Source: CAD feature listing. Evaluate the final solid. Frame: model axes, mm. A direction names the side the tool comes from. Round coordinates to 2 decimals unless told otherwise and drop trailing zeros. Write each loop counter-clockwise with the first axis right and the second up, starting at its lowest first coordinate (ties: lowest second). Pieces come first, ordered by that corner, then holes.
from build123d import *

# Parameters (mm, degrees)
SKETCH1_W               = 38.1
SKETCH1_H               = 19.05
BOSS_EXTRUDE1_DEPTH     = 12.7
SKETCH2_W               = 11.43
SKETCH2_H               = 19.05
CUT_EXTRUDE1_DEPTH      = 20.05
SKETCH3_R               = 3.302
CUT_EXTRUDE2_DEPTH      = 7.35
SKETCH7_R               = 6.35
CUT_EXTRUDE6_DEPTH      = 19.05
F_1_4_20_TAPPED_HOLE2_D = 5.1054


with BuildPart() as part:
    # Sketch1 → Boss-Extrude1 (new body, symmetric)
    with BuildSketch(Plane(origin=(0, 0, 0), x_dir=(1, 0, 0), z_dir=(0, 1, 0))):
        Rectangle(SKETCH1_W, SKETCH1_H)
    extrude(amount=BOSS_EXTRUDE1_DEPTH, both=True)

    # Sketch2 → Cut-Extrude1 (cut, through all)
    with BuildSketch(Plane.XY.offset(9.525)):
        with Locations((-13.335, 3.175)):
            Rectangle(SKETCH2_W, SKETCH2_H)
    cut_extrude1 = extrude(amount=-CUT_EXTRUDE1_DEPTH, mode=Mode.SUBTRACT)

    # Sketch3 → Cut-Extrude2 (cut, through all)
    with BuildSketch(Plane(origin=(0, -6.35, 0), x_dir=(1, 0, 0), z_dir=(0, 1, 0))):
        with Locations((-12.7, 0)):
            Circle(SKETCH3_R)
    cut_extrude2 = extrude(amount=-CUT_EXTRUDE2_DEPTH, mode=Mode.SUBTRACT)

    # Mirror1: Cut-Extrude1, Cut-Extrude2 across plane
    add(cut_extrude1.mirror(Plane(origin=(0, 0, 0), x_dir=(0, 0, 1), z_dir=(1, 0, 0))), mode=Mode.SUBTRACT)
    add(cut_extrude2.mirror(Plane(origin=(0, 0, 0), x_dir=(0, 0, 1), z_dir=(1, 0, 0))), mode=Mode.SUBTRACT)

    # Sketch7 → Cut-Extrude6 (cut)
    with BuildSketch(Plane.XZ.offset(12.7)):
        Circle(SKETCH7_R)
    extrude(amount=-CUT_EXTRUDE6_DEPTH, mode=Mode.SUBTRACT)

    # 1/4-20 Tapped Hole2 (through all)
    with Locations(Plane(origin=(0, 12.7, 0), x_dir=(1, 0, 0), z_dir=(0, 1, 0))):
        with Locations((0, 0)):
            Hole(F_1_4_20_TAPPED_HOLE2_D / 2)


solid = part.part
1) Pull-direction query (Z, two-part tool) for faces 4 (the face through (-2.435, 9.481, -0.767)), 5 (the face through (0, -3, -9.525)), 6 (the face through (19.05, -9, 0)); classes: released by +Z, released by -Z, zero draft, split by the parting line, or undercut.
Taken from the geometry:
face 4: undercut
face 5: released by -Z
face 6: zero draft
2) Section query A-A on x = 0. Return the cut outline in (y, z) (3 decimals), then the cut area to 3 significant figures.
Taken from the geometry:
outline: (-12.7, -9.525) - (12.7, -9.525) - (12.7, -2.553) - (6.35, -2.553) - (6.35, -6.35) - (-12.7, -6.35) - close; (-12.7, 6.35) - (6.35, 6.35) - (6.35, 2.553) - (12.7, 2.553) - (12.7, 9.525) - (-12.7, 9.525) - close
area: 210 mm2
3) Material intervals for line 1 (Z direction, x = 12.7, y = -9.5) (3 decimals); line 2 (Z direction, x = 0, y = 10) (3 decimals); line 3 (Y direction, x = -12, z = -7), sorted ascending.
Taken from the geometry:
line 1: z = -9.525 to -3.302, 3.302 to 9.525
line 2: z = -9.525 to -2.553, 2.553 to 9.525
line 3: y = -12.7 to -6.35
4) Section query D-D on x = -12.7. Return the cut outline in (y, z) (3 decimals), then the cut area to 3 significant figures.
Taken from the geometry:
outline: (-12.7, -9.525) - (-6.35, -9.525) - (-6.35, -3.302) - (-12.7, -3.302) - close; (-12.7, 3.302) - (-6.35, 3.302) - (-6.35, 9.525) - (-12.7, 9.525) - close
area: 79.0 mm2
5) Contact query for flat-ended pins moving along their axis: P1, Ø1.5, axis at y = -5, z = -5.5, coming from the +X side; P2, Ø7.5, axis at x = -12.7, z = 0, coming from the +Y side; P3, Ø2, axis at y = -2, z = -2, coming from the -X side. Output: stop coordinate, or through.
Taken from the geometry:
P1: stops at x = 7.62
P2: stops at y = -6.35
P3: stops at x = -7.62
6) Reachability of faces 1 (the face through (3, 6.35, 0)), 2 (the face through (7.62, 3, 0)), 3 (the face through (-7.62, 3, 0)) from +Z, -Z, +X, -X, +Y, -Y: full face, straight path, thin tool, end or side. Return the list, or none.
Taken from the geometry:
face 1: -Y
face 2: +Z, -Z, +X, +Y
face 3: +Z, -Z, -X, +Y
7) Section query B-B on y = 7.5. Return the cut outline in (x, z) (3 decimals).
Taken from the geometry:
outline: (-7.62, -9.525) - (7.62, -9.525) - (7.62, 9.525) - (-7.62, 9.525) - close; hole circle Ø5.105 at (0, 0)
8) Section query C-C on z = 0. Return the cut outline in (x, y), then the cut area to 3 significant figures.
Taken from the geometry:
outline: (-19.05, -12.7) - (-16, -12.7) - (-16, -6.35) - (-19.05, -6.35) - close; (-9.4, -12.7) - (-6.35, -12.7) - (-6.35, 6.35) - (-2.55, 6.35) - (-2.55, 12.7) - (-7.62, 12.7) - (-7.62, -6.35) - (-9.4, -6.35) - close; (2.55, 6.35) - (6.35, 6.35) - (6.35, -12.7) - (9.4, -12.7) - (9.4, -6.35) - (7.62, -6.35) - (7.62, 12.7) - (2.55, 12.7) - close; (16, -12.7) - (19.05, -12.7) - (19.05, -6.35) - (16, -6.35) - close
area: 174 mm2
